from build123d import *

# Parameters (mm, degrees)
SKETCH1_R               = 1.5
BOSS_EXTRUDE1_DEPTH     = 105
FILLET1_R               = 10
CUT_EXTRUDE1_DEPTH      = 117.542660484
CUT_EXTRUDE1_DEPTH_BACK = 117.542660484
CAVITY1_DEPTH           = 3
SKETCH3_R               = 2.5
SKETCH3_R_2             = 1.5
BOSS_EXTRUDE2_DEPTH     = 20
SKETCH5_R               = 1.5
BOSS_EXTRUDE4_DEPTH     = 37
BOSS_EXTRUDE5_START     = -62
SKETCH5_2_R             = 1.5
BOSS_EXTRUDE5_DEPTH     = 40


# Read off the part's stored shape, not the designer's step: Cavity1
with BuildPart() as part:
    # Sketch1 → Boss-Extrude1 (new body)
    with BuildSketch(Plane(origin=(0, 0, 0), x_dir=(0, 0, -1), z_dir=(1, 0, 0))):
        with BuildLine():
            add(Edge.make_bspline(
                [(3.73e-07, 7.5), (-15, 0), (-3.73e-07, -7.5)],
                knots=[0, 0, 0, 1, 1, 1], degree=2, weights=[1, 2.333333333, 1]))
            add(Edge.make_bspline(
                [(3.73e-07, 7.5), (100, 0), (-3.73e-07, -7.5)],
                knots=[0, 0, 0, 1, 1, 1], degree=2, weights=[1, 1.001467765, 1]))
        make_face()
        Circle(SKETCH1_R, mode=Mode.SUBTRACT)
    extrude(amount=BOSS_EXTRUDE1_DEPTH)

    # Fillet1
    fillet1_edges = [part.edges().sort_by_distance(p)[0] for p in [
        (52.5, -7.5, 3.73e-07),
        (52.5, 7.5, -3.73e-07),
    ]]
    fillet(fillet1_edges, radius=FILLET1_R)

    # Sketch2 → Cut-Extrude1 (cut, two sides: drawn at the far end of the back side and taken through both)
    with BuildSketch(Plane(origin=(0, 0, 0), x_dir=(1, 0, 0), z_dir=(0, 1, 0)).offset(-CUT_EXTRUDE1_DEPTH_BACK)):
        with BuildLine():
            Line((65, 19.76833361), (65, 24.578179161))
            ThreePointArc((65, 24.578179161), (52.5, 34.902500415), (40, 24.578179161))
            Line((40, 24.578179161), (40, 19.76833361))
            Line((40, 19.76833361), (40, 14.958488059))
            ThreePointArc((40, 14.958488059), (52.5, 4.634166805), (65, 14.958488059))
            Line((65, 14.958488059), (65, 19.76833361))
        make_face()
        with BuildLine():
            Line((40, -10.5), (65, -10.5))
            Line((65, -10.5), (65, 14.958488059))
            ThreePointArc((65, 14.958488059), (52.5, 4.634166805), (40, 14.958488059))
            Line((40, 14.958488059), (40, -10.5))
        make_face()
    extrude(amount=CUT_EXTRUDE1_DEPTH + CUT_EXTRUDE1_DEPTH_BACK, mode=Mode.SUBTRACT)

    # Cavity1 outline → Cavity1 (cut)
    with BuildSketch(Plane.YZ):
        with BuildLine():
            ThreePointArc((-2, -13.75), (0, -15.75), (2, -13.75))
            Line((2, -13.75), (2.497863905, -2.796994085))
            ThreePointArc((2.497863905, -2.796994085), (0, 3.75), (-2.497863905, -2.796994085))
            Line((-2.497863905, -2.796994085), (-2, -13.75))
        make_face()
    extrude(amount=CAVITY1_DEPTH, mode=Mode.SUBTRACT)

    # Sketch3 → Boss-Extrude2 (add)
    # profile 1 of 2: a face of its own
    with BuildSketch(Plane(origin=(105, 0, 0), x_dir=(0, 0, -1), z_dir=(1, 0, 0))):
        Circle(SKETCH3_R)
        with Locations(Location((0, 0, 0), (0, 0, 180))):
            Circle(SKETCH3_R_2, mode=Mode.SUBTRACT)
    # profile 2 of 2: a face of its own
    with BuildSketch(Plane(origin=(105, 0, 0), x_dir=(0, 0, -1), z_dir=(1, 0, 0))):
        with Locations(Location((0, 0, 0), (0, 0, 180))):
            Circle(SKETCH3_R_2)
    extrude(amount=BOSS_EXTRUDE2_DEPTH)

    # Sketch5 → Boss-Extrude4 (add)
    with BuildSketch(Plane.ZY.offset(-3)):
        with Locations(Location((0, 0, 0), (0, 0, 180))):
            Circle(SKETCH5_R)
    extrude(amount=-BOSS_EXTRUDE4_DEPTH)

    # Sketch5<2> → Boss-Extrude5 (add)
    with BuildSketch(Plane.ZY.offset(-3).offset(BOSS_EXTRUDE5_START)):
        Circle(SKETCH5_2_R)
    extrude(amount=-BOSS_EXTRUDE5_DEPTH)


solid = part.part
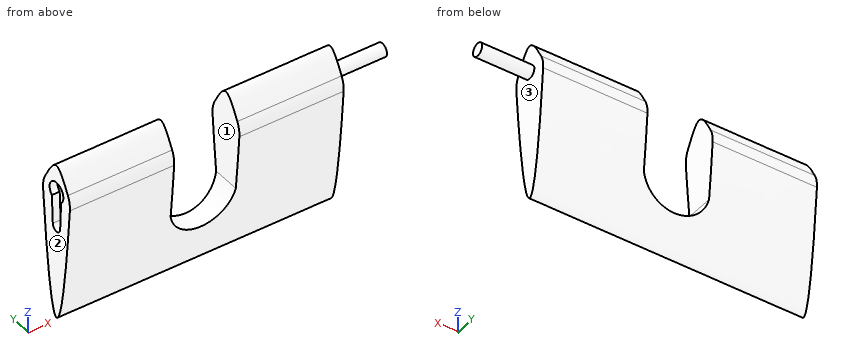
The listing builds one solid part. Answer for the finished solid, in the listing's coordinates (mm). Face numbers are marked on the shaded views. Give positions to 0.01 mm unless a question says otherwise; leave off trailing zeros. Write each loop counter-clockwise with the first axis right and the second up, starting at its lowest first coordinate (ties: lowest second). Pieces come first, ordered by that corner, then holes.
Item 1: Find the intervals of material crossed by line 1 along X through (y, z) = (-5.25, -10.5); line 2 along Z through (x, y) = (1.5, 0); line 3 along X through (y, z) = (2, 1), in increasing order.
Item 2: Determine the mould class of the marked faces 1, 2 and 3 for opening direction X: released by +X, released by -X, zero draft, split by the parting line, or undercut.
Item 3: Flat-ended cylindrical pins translate along their axes: P1, Ø5, axis at y = 2.5, z = -15, coming from the +X side; P2, Ø2, axis at x = 19, z = -24.5, coming from the +Y side; P3, Ø3, axis at x = 39.5, y = -3.5, coming from the +Z side; P4, Ø6, axis at x = 61.5, z = -9, coming from the -Y side. Find the tip coordinate at first contact, or state that the pin passes through.
Item 4: Section A-A, the plane x = 114.5 is taken. Write down the section's boundary in (y, z), plus the area to 3 significant figures.
Completed:
1. line 1: x = 0 to 40, 65 to 105
1. line 2: z = -50.04 to -15.75, 3.75 to 10.5
1. line 3: x = 3 to 40, 65 to 125
2. face 1: undercut
2. face 2: released by -X
2. face 3: released by +X
3. P1: stops at x = 105
3. P2: stops at y = 5.46
3. P3: stops at z = 9.34
3. P4: passes through
4. outline: circle Ø5 at (0, 0)
4. area: 19.6 mm2
